Input: dimensioned drawing with shaded views. Units: mm. Origin: part minimum x, y, z. Coordinates: 2 decimals unless noted, no trailing zeros. Write each loop counter-clockwise with the first axis right and the second up, starting at its lowest first coordinate (ties: lowest second). Pieces come first, ordered by that corner, then holes. Notation, with made-up numbers: (-33, 29) -> (-5, 29) arc R23 cw to (-5, 55) -> close; hole circle Ø9 at (74, 16.5). An arc over 180 degrees is marked (long way). One line per item, written item: value. Start each with the question number.
1. First-contact query: P1, Ø1, axis at x = 1, z = 3.5, coming from the +Y side; P2, Ø1.2, axis at x = 3.5, y = 3.5, coming from the +Z side; P3, Ø2, axis at y = 5, z = 3, coming from the +X side; P4, Ø3, axis at x = 1.5, y = 2.5, coming from the +Z side. Flat tips, straight axial feed; report the tip coordinate or a pass-through.
2. Mould query, pull axis X, two halves, no side actions, for the marked faces 1, 2, 3 and 4. Classes: released by +X, released by -X, zero draft, split by the parting line, or undercut.
3. Section query C-C, the plane z = 2.2. Output: boundary loops of the cut face in (x, y).
4. Section query A-A, the plane y = 3. Output: boundary loops of the cut face in (x, z).
5. Section query D-D, the plane z = 0.3. Output: boundary loops of the cut face in (x, y), and give its area (3 significant figures).
6. Line query: line 1 (Y direction, x = 3, z = 3.1); line 2 (Z direction, x = 2.1, y = 4.35); line 3 (X direction, y = 3.9, z = 1.35). Output: solid intervals per line, ascending.
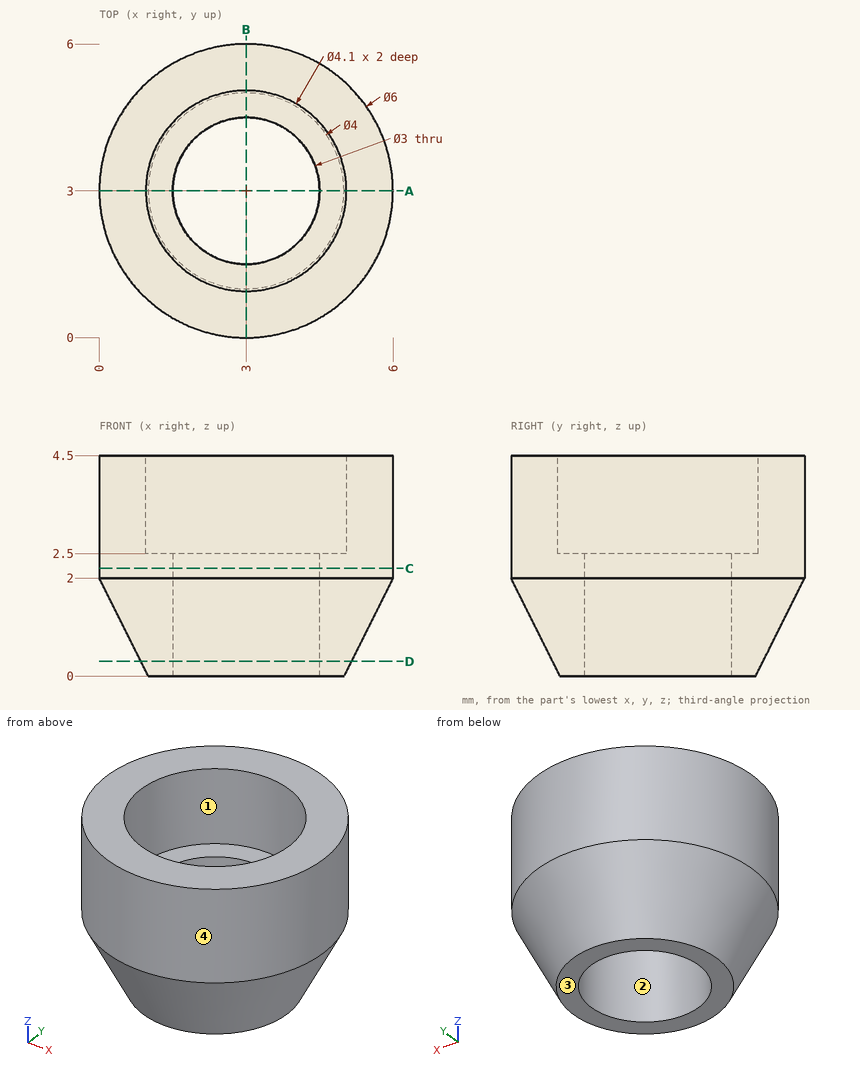
Computed values:
1. P1: stops at y = 5.6
1. P2: passes through
1. P3: stops at x = 5.83
1. P4: stops at z = 4.5
2. face 1: undercut
2. face 2: undercut
2. face 3: zero draft
2. face 4: split by the parting line
3. outline: circle Ø6 at (3, 3); hole circle Ø3 at (3, 3)
4. outline: (0, 2) -> (1, 0) -> (1.5, 0) -> (1.5, 2.5) -> (0.95, 2.5) -> (0.95, 4.5) -> (0, 4.5) -> close; (4.5, 0) -> (5, 0) -> (6, 2) -> (6, 4.5) -> (5.05, 4.5) -> (5.05, 2.5) -> (4.5, 2.5) -> close
5. outline: circle Ø4.3 at (3, 3); hole circle Ø3 at (3, 3)
5. area: 7.45 mm²
6. line 1: y = 0 to 0.95, 5.05 to 6
6. line 2: z = 0 to 2.5
6. line 3: x = 0.48 to 1.8, 4.2 to 5.52
